from build123d import *

# Parameters (mm, degrees)
SKETCH1_W           = 72.5
SKETCH1_H           = 45.5
SKETCH1_R           = 1.75
SKETCH1_W_2         = 37
SKETCH1_H_2         = 21.5
BOSS_EXTRUDE1_DEPTH = 3


with BuildPart() as part:
    # Sketch1 → Boss-Extrude1 (new body)
    with BuildSketch(Plane(origin=(0, 0, 0), x_dir=(1, 0, 0), z_dir=(0, 1, 0))):
        with Locations((36.25, 22.75)):
            Rectangle(SKETCH1_W, SKETCH1_H)
        with Locations((68.5, 22.75)):
            Circle(SKETCH1_R, mode=Mode.SUBTRACT)
        with Locations((4, 41.5)):
            Circle(SKETCH1_R, mode=Mode.SUBTRACT)
        with Locations((4, 4)):
            Circle(SKETCH1_R, mode=Mode.SUBTRACT)
        with Locations((36.25, 22.75)):
            Rectangle(SKETCH1_W_2, SKETCH1_H_2, mode=Mode.SUBTRACT)
    extrude(amount=BOSS_EXTRUDE1_DEPTH)


solid = part.part
The listing builds one solid part. Answer for the finished solid, in the listing's coordinates (mm). A direction names the side the tool comes from. Coordinates: 2 decimals unless noted, no trailing zeros. Write each loop counter-clockwise with the first axis right and the second up, starting at its lowest first coordinate (ties: lowest second). Pieces come first, ordered by that corner, then holes. Notation, with made-up numbers: M 77.5,28 L 115.5,28 A25 ccw 115.5,66 Z; hole C -25.75,58 d10. An arc over 180 degrees is marked long. Put each result on its own line as item: value. Start each with the question number.
1. A cutting plane is placed at D-D on x = 4. Write down the section's boundary in (y, z).
2. A cutting plane is placed at A-A on z = -41.5. Write down the section's boundary in (x, y).
3. Which of the six approach directions +Z, -Z, +X, -X, +Y, -Y give full straight-line access (tool end or side, diameter ignored) to faces 1 (the flat face through (36, 1, -33.5)), 2 (the flat face through (72.5, 1, -22))?
4. A flat-ended cylindrical pin translates along its axis: P1, Ø1, axis at x = 37.5, z = -31.5, coming from the +Y side. Find the tip coordinate at first contact, or state that the pin passes through.
5. For a pull along Z with two mould halves and no side action, classify faces 3 (the flat face through (36, 0, -38)), 4 (the flat face through (36, 1, -45.5)), 5 (the flat face through (36, 1, -12)), 6 (the flat face through (36, 1, 0)) as pulls with the +Z half, pulls with the -Z half, needs draft (parallel to the pull), parting line crosses it, or undercut.
6. Consider line 1 (Z direction, x = 4, y = 1); line 2 (X direction, y = 0.95, z = -22.75); line 3 (X direction, y = 1, z = -16). Determine where each line is inside the solid, lowest interval first. Write a range as from..to.
7. A cutting plane is placed at C-C on x = 23. Write down the section's boundary in (y, z).
8. A cutting plane is placed at B-B on y = 1.35. Write down the section's boundary in (x, z), then the cut area to 3 significant figures.
Resolved:
1. outline: M 0,-45.5 L 3,-45.5 L 3,-43.25 L 0,-43.25 Z; M 0,-39.75 L 3,-39.75 L 3,-5.75 L 0,-5.75 Z; M 0,-2.25 L 3,-2.25 L 3,0 L 0,0 Z
2. outline: M 0,0 L 2.25,0 L 2.25,3 L 0,3 Z; M 5.75,0 L 72.5,0 L 72.5,3 L 5.75,3 Z
3. face 1: +Y, -Y
3. face 2: +Z, -Z, +X, +Y, -Y
4. P1: passes through
5. face 3: needs draft
5. face 4: pulls with the -Z half
5. face 5: undercut
5. face 6: pulls with the +Z half
6. line 1: z = -45.5..-43.25, -39.75..-5.75, -2.25..0
6. line 2: x = 0..17.75, 54.75..66.75, 70.25..72.5
6. line 3: x = 0..17.75, 54.75..72.5
7. outline: M 0,-45.5 L 3,-45.5 L 3,-33.5 L 0,-33.5 Z; M 0,-12 L 3,-12 L 3,0 L 0,0 Z
8. outline: M 0,-45.5 L 72.5,-45.5 L 72.5,0 L 0,0 Z; hole C 4,-41.5 d3.5; hole C 4,-4 d3.5; hole M 17.75,-33.5 L 54.75,-33.5 L 54.75,-12 L 17.75,-12 Z; hole C 68.5,-22.75 d3.5
8. area: 2,470 mm2
